```python
from build123d import *

# Parameters (mm, degrees)
F0_W     = 320.04
F0_H     = 320.04
F1_DEPTH = 32.385
F2_W     = 309.88
F2_H     = 309.88
F3_DEPTH = 28.575
F4_W     = 5.08
F4_H     = 309.88
F5_DEPTH = 5.08


with BuildPart() as f1:
    # F0 (on Top) → F1 (new body)
    with BuildSketch(Plane.XY):
        Rectangle(F0_W, F0_H)
    extrude(amount=F1_DEPTH)

    # F2 (on face) → F3 (cut)
    with BuildSketch(Plane.XY.offset(32.385)):
        Rectangle(F2_W, F2_H)
    extrude(amount=-F3_DEPTH, mode=Mode.SUBTRACT)

    # F4 (on face) → F5 (cut)
    with BuildSketch(Plane.XY.offset(32.385)):
        with Locations((157.48, 0)):
            Rectangle(F4_W, F4_H)
    extrude(amount=-F5_DEPTH, mode=Mode.SUBTRACT)


solid = f1.part
```
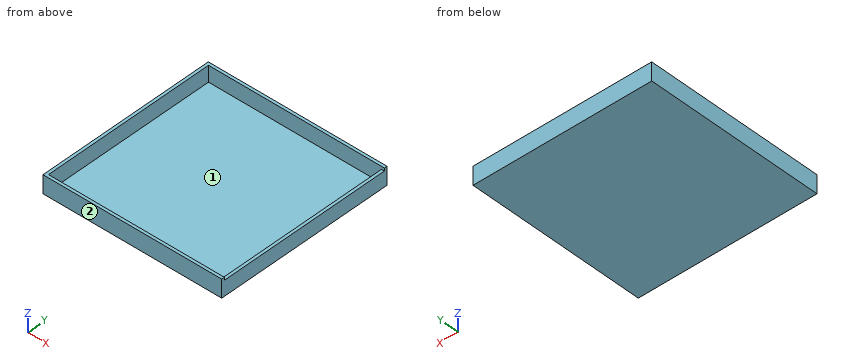
CAD build for the part. Positions are in the model's coordinates, mm. Face numbers are marked on the shaded views. Coordinates: 2 decimals unless noted, no trailing zeros. Order: outer loops, then holes, each group sorted by start corner. A loop starts at its lowest first (then second) coordinate and runs counter-clockwise, first axis right, second up. Notation, with made-up numbers: (26.25, -2) -> (72.25, -2) arc R29 cw to (72.25, 28) -> close; hole circle Ø5 at (49.25, 41.5). An arc over 180 degrees is marked (long way). Use one line per item in the form item = value. Start each with the question number.
1) Band-saw the part on A-A on z = 23. Give the cut face in (x, y).
2) Pull direction X, two halves, no side cores. Call the marked faces 1 and 2: +X half, -X half, draft (parallel to the pull), parting line (faces both ways), or undercut.
3) Band-saw the part on C-C on x = 14. Give the cut face in (y, z) (3 decimals).
4) Band-saw the part on B-B on y = -138. Give the cut face in (x, z) (3 decimals), then the cut area to 3 significant figures.
5) Drill centre lines: L1, parallel to X at y = -19.5, z = 5; L2, parallel to Z at x = 92, y = 20. Where is each one in solid material? Low to high. Write a range as [from, to].
6) Drop flat-ended pins along their axis: pin 1 (4 mm diameter, centred on x = 3.5, y = -70.5, fed in from -Z); pin 2 (4 mm diameter, centred on x = 158, y = -31.5, fed in from +Z) (3 decimals). Give the stop position or say it passes through.
Entries:
q1.outline = (-160.02, -160.02) -> (160.02, -160.02) -> (160.02, 160.02) -> (-160.02, 160.02) -> close; hole (-154.94, -154.94) -> (154.94, -154.94) -> (154.94, 154.94) -> (-154.94, 154.94) -> close
q2.face_1 = undercut
q2.face_2 = draft
q3.outline = (-160.02, 0) -> (160.02, 0) -> (160.02, 32.385) -> (154.94, 32.385) -> (154.94, 3.81) -> (-154.94, 3.81) -> (-154.94, 32.385) -> (-160.02, 32.385) -> close
q4.outline = (-160.02, 0) -> (160.02, 0) -> (160.02, 27.305) -> (154.94, 27.305) -> (154.94, 3.81) -> (-154.94, 3.81) -> (-154.94, 32.385) -> (-160.02, 32.385) -> close
q4.area = 1,480 mm2
q5.L1 = [-160.02, -154.94], [154.94, 160.02]
q5.L2 = [0, 3.81]
q6.pin_1 = 0
q6.pin_2 = 27.305
